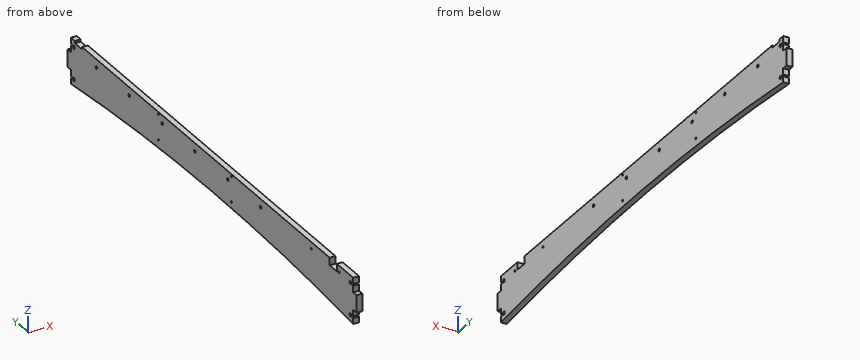
from build123d import *

# Parameters (mm, degrees)
DODANIE_WYCI_GNI_CIE1_DEPTH = 10
SZKIC1_W                    = 30
SZKIC1_H                    = 10.1
SZKIC1_W_2                  = 25
WYTNIJ_WYCI_GNI_CIE1_DEPTH  = 10
WYTNIJ_WYCI_GNI_CIE2_DEPTH  = 10
SZYK_LINIOWY1_COUNT         = 2
SZYK_LINIOWY1_PITCH         = 55
SZKIC5_R                    = 1.55
WYTNIJ_WYCI_GNI_CIE3_DEPTH  = 10
SZKIC7_R                    = 2.45
WYTNIJ_WYCI_GNI_CIE5_DEPTH  = 10
SZYK_LINIOWY3_COUNT         = 6
SZYK_LINIOWY3_PITCH         = 100
SZKIC8_W                    = 13
SZKIC8_H                    = 22
WYTNIJ_WYCI_GNI_CIE6_DEPTH  = 10
SZKIC9_W                    = 4
SZKIC9_H                    = 22
WYTNIJ_WYCI_GNI_CIE7_DEPTH  = 10
LUSTRO1_COPY_1_DEPTH        = 10
SZKIC12_R                   = 1.55
WYTNIJ_WYCI_GNI_CIE8_DEPTH  = 10
SZYK_LINIOWY4_COUNT         = 2
SZYK_LINIOWY4_PITCH         = 223


with BuildPart() as part:
    # Szkic11 → Dodanie-wyciągnięcie1 (new body)
    with BuildSketch(Plane.ZY.offset(-248.52281754)):
        with BuildLine():
            Line((-79.001367167, 0), (0, 0))
            Line((0, 0), (0, 880))
            Line((0, 880), (-78.955177412, 880))
            Line((-78.955177412, 880), (-78.955177412, 870))
            ThreePointArc((-78.955177412, 870), (-57.819766969, 439.998863597), (-79.001367167, 10))
            Line((-79.001367167, 10), (-79.001367167, 0))
        make_face()
    extrude(amount=DODANIE_WYCI_GNI_CIE1_DEPTH)

    # Szkic1 → Wytnij-wyciągnięcie1 (cut)
    with BuildSketch(Plane(origin=(248.52281754, 0, 0), x_dir=(0, 0, -1), z_dir=(1, 0, 0))):
        with Locations((70, 874.95)):
            Rectangle(SZKIC1_W, SZKIC1_H)
        with Locations((12.5, 874.95)):
            Rectangle(SZKIC1_W_2, SZKIC1_H)
    wytnij_wyci_gni_cie1 = extrude(amount=-WYTNIJ_WYCI_GNI_CIE1_DEPTH, mode=Mode.SUBTRACT)

    # Szkic2 → Wytnij-wyciągnięcie2 (cut)
    with BuildSketch(Plane(origin=(248.52281754, 0, 0), x_dir=(0, 0, -1), z_dir=(1, 0, 0))):
        Polygon((10.660920663, 869.9), (13.760920663, 869.9), (13.760920663, 861.4), (15.135920663, 861.4), (15.135920663, 859.4), (13.760920663, 859.4), (13.760920663, 858.9), (10.660920663, 858.9), (10.660920663, 859.4), (9.285920663, 859.4), (9.285920663, 861.4), (10.660920663, 861.4), align=None)
    wytnij_wyci_gni_cie2 = extrude(amount=-WYTNIJ_WYCI_GNI_CIE2_DEPTH, mode=Mode.SUBTRACT)

    # Szyk liniowy1: Wytnij-wyciągnięcie2 ×2
    with Locations(*[(0, 0, -i * SZYK_LINIOWY1_PITCH) for i in range(1, SZYK_LINIOWY1_COUNT)]):
        add(wytnij_wyci_gni_cie2, mode=Mode.SUBTRACT)

    # Szkic5 → Wytnij-wyciągnięcie3 (cut)
    with BuildSketch(Plane.ZY.offset(-248.52281754)):
        with Locations((-11.55, 53)):
            Circle(SZKIC5_R)
        with Locations((-11.55, 138)):
            Circle(SZKIC5_R)
    extrude(amount=WYTNIJ_WYCI_GNI_CIE3_DEPTH, mode=Mode.SUBTRACT)

    # Szkic7 → Wytnij-wyciągnięcie5 (cut)
    with BuildSketch(Plane(origin=(248.52281754, 0, 0), x_dir=(0, 0, -1), z_dir=(1, 0, 0))):
        with Locations((14.31069395, 792.236985413)):
            Circle(SZKIC7_R)
    wytnij_wyci_gni_cie5 = extrude(amount=-WYTNIJ_WYCI_GNI_CIE5_DEPTH, mode=Mode.SUBTRACT)

    # Szyk liniowy3: Wytnij-wyciągnięcie5 ×6
    with Locations(*[(0, -i * SZYK_LINIOWY3_PITCH, 0) for i in range(1, SZYK_LINIOWY3_COUNT)]):
        add(wytnij_wyci_gni_cie5, mode=Mode.SUBTRACT)

    # Szkic8 → Wytnij-wyciągnięcie6 (cut)
    with BuildSketch(Plane(origin=(248.52281754, 0, 0), x_dir=(0, 0, -1), z_dir=(1, 0, 0))):
        with Locations((6.5, 71)):
            Rectangle(SZKIC8_W, SZKIC8_H)
    extrude(amount=-WYTNIJ_WYCI_GNI_CIE6_DEPTH, mode=Mode.SUBTRACT)

    # Szkic9 → Wytnij-wyciągnięcie7 (cut)
    with BuildSketch(Plane(origin=(248.52281754, 0, 0), x_dir=(0, 0, -1), z_dir=(1, 0, 0))):
        with Locations((2, 846.9)):
            Rectangle(SZKIC9_W, SZKIC9_H)
    extrude(amount=-WYTNIJ_WYCI_GNI_CIE7_DEPTH, mode=Mode.SUBTRACT)

    # Lustro1: Wytnij-wyciągnięcie1, Wytnij-wyciągnięcie2 across plane
    add(wytnij_wyci_gni_cie1.mirror(Plane.ZX.offset(440)), mode=Mode.SUBTRACT)
    add(wytnij_wyci_gni_cie2.mirror(Plane.ZX.offset(440)), mode=Mode.SUBTRACT)

    # Lustro1 copy 1 sketch → Lustro1 copy 1 (cut)
    with BuildSketch(Plane(origin=(248.52281754, 880, -55), x_dir=(0, 0, -1), z_dir=(1, 0, 0))):
        Polygon((10.660920663, -869.9), (13.760920663, -869.9), (13.760920663, -861.4), (15.135920663, -861.4), (15.135920663, -859.4), (13.760920663, -859.4), (13.760920663, -858.9), (10.660920663, -858.9), (10.660920663, -859.4), (9.285920663, -859.4), (9.285920663, -861.4), (10.660920663, -861.4), align=None)
    extrude(amount=-LUSTRO1_COPY_1_DEPTH, mode=Mode.SUBTRACT)

    # Szkic12 → Wytnij-wyciągnięcie8 (cut)
    with BuildSketch(Plane.ZY.offset(-238.52281754)):
        with Locations((-47.7, 603.736985413)):
            Circle(SZKIC12_R)
        with Locations((-3.7, 603.736985413)):
            Circle(SZKIC12_R)
    wytnij_wyci_gni_cie8 = extrude(amount=-WYTNIJ_WYCI_GNI_CIE8_DEPTH, mode=Mode.SUBTRACT)

    # Szyk liniowy4: Wytnij-wyciągnięcie8 ×2
    with Locations(*[(0, -i * SZYK_LINIOWY4_PITCH, 0) for i in range(1, SZYK_LINIOWY4_COUNT)]):
        add(wytnij_wyci_gni_cie8, mode=Mode.SUBTRACT)


solid = part.part
Read the model definition and answer for the solid it produces. Units are mm, in the model's axes. Give positions to 0.01 mm unless a question says otherwise; leave off trailing zeros. Loops run counter-clockwise (first coordinate to the right, second up) from the corner with the lowest first, then second, coordinate; pieces in that order, holes last. Notation, with made-up numbers: M -1.75,44.5 L 29.25,44.5 A14 ccw 29.25,67.5 Z; hole C -33,-13.5 d3. An arc over 180 degrees is marked long. Write each question's results on one line, items separated by ' | '.
1. Straight lines are drawn through the part: line 1 (Y direction, x = 244, z = -11.55); line 2 (Y direction, x = 242, z = -3.7); line 3 (Y direction, x = 241.25, z = -47.7). For each, find the intervals that lie inside material, in ascending order. Write a range as [from, to].
Values:
line 1: y = [21.1, 51.45], [54.55, 60], [82, 136.45], [139.55, 858.9] | line 2: y = [10.1, 60], [82, 379.19], [382.29, 602.19], [605.29, 835.9], [857.9, 869.9] | line 3: y = [0, 379.19], [382.29, 602.19], [605.29, 880]
2. Given pin 1 (6 mm diameter, centred on x = 241.5, z = -8.5, fed in from +Y); pin 2 (3 mm diameter, centred on x = 244, z = -59, fed in from -Y); pin 3 (2 mm diameter, centred on x = 242, y = 860.5, fed in from -Z), each flat-ended and moving along its own axis, determine where each tip first touches the part or whether it passes through.
Values:
pin 1: stops at y = 869.9 | pin 2: stops at y = 10.1 | pin 3: stops at z = -78.13
3. Section A-A on y = 358 is taken. Give the vertices of the cut face in (x, z).
Values:
outline: M 238.52,-58.59 L 248.52,-58.59 L 248.52,0 L 238.52,0 Z
4. Section B-B on x = 243.25 is taken. State how many separate pieces and enclosed holes the cut face has, plus the area to 3 significant figures.
Values:
separate pieces: 1 | enclosed holes: 12 | area: 55,700 mm^2
5. Section C-C on y = 477 is taken. Give the vertices of the cut face in (x, z), plus the area to 3 significant figures.
Values:
outline: M 238.52,-57.97 L 248.52,-57.97 L 248.52,0 L 238.52,0 Z | area: 580 mm^2
